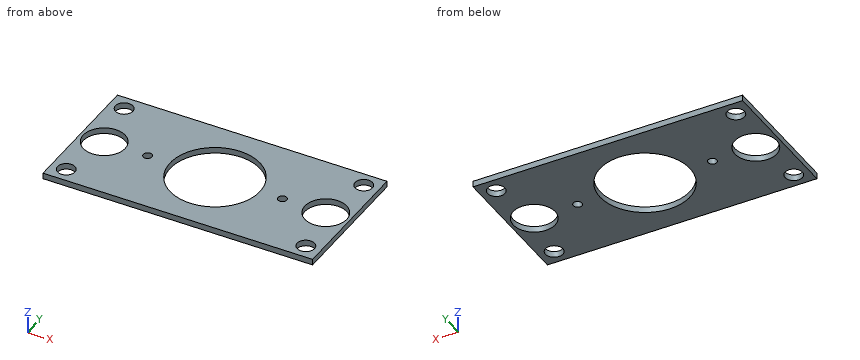
```python
from build123d import *

# Parameters (mm, degrees)
SKETCH_1_W      = 90
SKETCH_1_H      = 45
SKETCH_1_R      = 2.9
SKETCH_1_R_2    = 1.45
SKETCH_1_R_3    = 15
SKETCH_1_R_4    = 7
EXTRUDE_2_DEPTH = 2


with BuildPart() as part:
    # 草图1 → 凸台-拉伸2 (new body)
    with BuildSketch(Plane.XY):
        Rectangle(SKETCH_1_W, SKETCH_1_H)
        with Locations((-40, 17.5)):
            Circle(SKETCH_1_R, mode=Mode.SUBTRACT)
        with Locations((-40, -17.5)):
            Circle(SKETCH_1_R, mode=Mode.SUBTRACT)
        with Locations((40, 17.5)):
            Circle(SKETCH_1_R, mode=Mode.SUBTRACT)
        with Locations((40, -17.5)):
            Circle(SKETCH_1_R, mode=Mode.SUBTRACT)
        with Locations((22.5, 0)):
            Circle(SKETCH_1_R_2, mode=Mode.SUBTRACT)
        with Locations((-22.5, 0)):
            Circle(SKETCH_1_R_2, mode=Mode.SUBTRACT)
        Circle(SKETCH_1_R_3, mode=Mode.SUBTRACT)
        with Locations((-37, 0)):
            Circle(SKETCH_1_R_4, mode=Mode.SUBTRACT)
        with Locations((37, 0)):
            Circle(SKETCH_1_R_4, mode=Mode.SUBTRACT)
    extrude(amount=-EXTRUDE_2_DEPTH)


solid = part.part
```
Could you check a few things on this model? Use its own coordinates, in mm. Round coordinates to 2 decimals unless told otherwise and drop trailing zeros. Loops run counter-clockwise (first coordinate to the right, second up) from the corner with the lowest first, then second, coordinate; pieces in that order, holes last. Notation, with made-up numbers: (1.5, 66) -> (51.5, 66) arc R20 cw to (51.5, 87) -> close; hole circle Ø2 at (-3, -7). An arc over 180 degrees is marked (long way). Put each result on its own line as item: value.
Q1. I want a section at D-D on x = -22.5. Write out the boundary of the cut face in (y, z), and give its area (3 significant figures).
Checks:
outline: (-22.5, -2) -> (-1.45, -2) -> (-1.45, 0) -> (-22.5, 0) -> close; (1.45, -2) -> (22.5, -2) -> (22.5, 0) -> (1.45, 0) -> close
area: 84.2 mm2
Q2. Please list where these lines run through material, in increasing order: line 1 (Y direction, x = 22.5, z = -1.05); line 2 (X direction, y = 18.5, z = -1.65); line 3 (X direction, y = 2.5, z = -0.65). Write a range as from..to.
Checks:
line 1: -22.5..-1.45, 1.45..22.5
line 2: -45..-42.72, -37.28..37.28, 42.72..45
line 3: -45..-43.54, -30.46..-14.79, 14.79..30.46, 43.54..45
Q3. I want a section at C-C on x = -40. Write out the boundary of the cut face in (y, z), and give its area (3 significant figures).
Checks:
outline: (-22.5, -2) -> (-20.4, -2) -> (-20.4, 0) -> (-22.5, 0) -> close; (-14.6, -2) -> (-6.32, -2) -> (-6.32, 0) -> (-14.6, 0) -> close; (6.32, -2) -> (14.6, -2) -> (14.6, 0) -> (6.32, 0) -> close; (20.4, -2) -> (22.5, -2) -> (22.5, 0) -> (20.4, 0) -> close
area: 41.5 mm2
Q4. I want a section at B-B on z = -0.5. Give the number of separate pieces and of enclosed holes in the cut face, and give its area (3 significant figures).
Checks:
separate pieces: 1
enclosed holes: 9
area: 2,920 mm2
Q5. I want a section at A-A on x = 0. Write out the boundary of the cut face in (y, z).
Checks:
outline: (-22.5, -2) -> (-15, -2) -> (-15, 0) -> (-22.5, 0) -> close; (15, -2) -> (22.5, -2) -> (22.5, 0) -> (15, 0) -> close
